from build123d import *

# Parameters (mm, degrees)
F1_DEPTH = 10
F3_DEPTH = 5
F5_DEPTH = 5
F6_W     = 56
F6_H     = 8
F6_W_2   = 46.4636435509
F6_H_2   = 28.4405329078
F7_DEPTH = 10


with BuildPart() as f1:
    # F0 (on Top) → F1 (new body)
    with BuildSketch(Plane.XY):
        Polygon((-156.0579602718, 94.9992052239), (-156.0579602718, -24.5707947761), (31.9420397282, -24.5707947761), (31.9420397282, 94.9992052239), (9.0120397282, 117.9292052239), (-133.1279602718, 117.9292052239), align=None)
    extrude(amount=F1_DEPTH)

    # F2 (on face) → F3 (cut)
    with BuildSketch(Plane.XY.offset(10)):
        Polygon((26.9420397282, 92.9281374121), (6.9409719163, 112.9292052239), (-131.05689246, 112.9292052239), (-151.0579602718, 92.9281374121), (-151.0579602718, -19.5707947761), (26.9420397282, -19.5707947761), align=None)
    extrude(amount=-F3_DEPTH, mode=Mode.SUBTRACT)

    # F4 (on face) → F5 (cut)
    with BuildSketch(Plane.XY.offset(5)):
        Polygon((-87.5216038227, 107.9292052239), (-87.5216038227, 69.2292052239), (-85.5216038227, 69.2292052239), (-85.5216038227, 107.9292052239), (-39.0579602718, 107.9292052239), (-39.0579602718, 69.2292052239), (-37.0579602718, 69.2292052239), (-37.0579602718, 107.9292052239), (-34.5216038227, 107.9292052239), (-34.5216038227, 109.9292052239), (-87.5216038227, 109.9292052239), (-90.5216038227, 109.9292052239), (-90.5216038227, 107.9292052239), align=None)
    extrude(amount=-F5_DEPTH, mode=Mode.SUBTRACT)

    # F6 (on face) → F7 (cut)
    with BuildSketch(Plane(origin=(0, 0, 0), x_dir=(1, 0, 0), z_dir=(0, 0, -1))):
        with Locations((-62.5216038227, -113.9292052239)):
            Rectangle(F6_W, F6_H)
        with Locations((-62.2897820473, -93.70893877)):
            Rectangle(F6_W_2, F6_H_2)
    extrude(amount=-F7_DEPTH, mode=Mode.SUBTRACT)


solid = f1.part
Work out the finished part from the listing and answer in its coordinate system (mm). A direction names the side the tool comes from. Coordinates: 2 decimals unless noted, no trailing zeros. Write each loop counter-clockwise with the first axis right and the second up, starting at its lowest first coordinate (ties: lowest second). Pieces come first, ordered by that corner, then holes. Notation, with made-up numbers: M 85.5,-37 L 97.5,-37 A17 cw 97.5,-27 Z; hole C 50.25,48 d9. An arc over 180 degrees is marked long. Answer as CSV lines item,"result". Start each with the question number.
Item 1: Consider L1, parallel to X at y = 84.5, z = 4.5; L2, parallel to X at y = 90, z = 8; L3, parallel to X at y = 72.5, z = 4.25. Determine where each line is inside the solid, lowest interval first.
Item 2: Section C-C on x = -99 is taken. Write down the section's boundary in (y, z).
Item 3: Section D-D on y = 62 is taken. Write down the section's boundary in (x, z).
Item 4: Section A-A on y = 88 is taken. Write down the section's boundary in (x, z).
Item 5: Section B-B on z = 8.25 is taken. Write down the section's boundary in (x, y), and give its area (3 significant figures).
Item 6: Determine the mould class of faces 1 (the face through (-63, -24.571, 5)), 2 (the face through (-63, 48, 5)), 3 (the face through (-63, 79.489, 2)) for opening direction Y: released by +Y, released by -Y, zero draft, split by the parting line, or undercut.
Item 7: A tool of negligible diameter and unlimited length cuts with its end or side. For faces 4 (the face through (-37.058, 88, 3)), 5 (the face through (-151.058, 37, 8)), 6 (the face through (31.942, 34, 5)), from which of +Z, -Z, +X, -X, +Y, -Y can it reach the whole face along a straight path? Write none if from no direction.
Item 8: Flat-ended cylindrical pins translate along their axes: P1, Ø12, axis at x = -23, y = 17.5, coming from the +Z side; P2, Ø0.9, axis at x = -89.5, z = 3, coming from the +Y side; P3, Ø1.5, axis at x = -71, z = 3, coming from the +Y side. Find the tip coordinate at first contact, or state that the pin passes through.
Checks:
1,L1,"x = -156.06 to -87.52, -37.06 to 31.94"
1,L2,"x = -156.06 to -151.06, 26.94 to 31.94"
1,L3,"x = -156.06 to -87.52, -85.52 to -39.06, -37.06 to 31.94"
2,outline,"M -24.57,0 L 117.93,0 L 117.93,10 L 112.93,10 L 112.93,5 L -19.57,5 L -19.57,10 L -24.57,10 Z"
3,outline,"M -156.06,0 L 31.94,0 L 31.94,10 L 26.94,10 L 26.94,5 L -151.06,5 L -151.06,10 L -156.06,10 Z"
4,outline,"M -156.06,0 L -87.52,0 L -87.52,5 L -151.06,5 L -151.06,10 L -156.06,10 Z; M -37.06,0 L 31.94,0 L 31.94,10 L 26.94,10 L 26.94,5 L -37.06,5 Z"
5,outline,"M -156.06,-24.57 L 31.94,-24.57 L 31.94,95 L 9.01,117.93 L -34.52,117.93 L -34.52,112.93 L 6.94,112.93 L 26.94,92.93 L 26.94,-19.57 L -151.06,-19.57 L -151.06,92.93 L -131.06,112.93 L -90.52,112.93 L -90.52,117.93 L -133.13,117.93 L -156.06,95 Z"
5,area,"2,800 mm²"
6,face 1,"released by -Y"
6,face 2,"undercut"
6,face 3,"released by +Y"
7,face 4,"+Z, -Z, +Y"
7,face 5,"+Z"
7,face 6,"+Z, -Z, +X, +Y, -Y"
8,P1,"stops at z = 5"
8,P2,"stops at y = 107.93"
8,P3,"stops at y = 79.49"
